```python
from build123d import *

# Parameters (mm, degrees)
EXTRUDE1_DEPTH = 0.4572
EXTRUDE2_REACH = 567.039
SKETCH2_R      = 6.35
EXTRUDE3_REACH = 567.039


with BuildPart() as part:
    # Sketch1 → Extrude1 (new body)
    with BuildSketch(Plane(origin=(0, 0, 0), x_dir=(1, 0, 0), z_dir=(0, 1, 0))):
        with BuildLine():
            Line((145.25625, 434.18125), (138.034060826, 516.73125))
            Line((138.034060826, 516.73125), (-138.034060826, 516.73125))
            Line((-138.034060826, 516.73125), (-145.25625, 434.18125))
            Line((-145.25625, 434.18125), (-228.6, 434.18125))
            Line((-228.6, 434.18125), (-228.6, 199.23125))
            Line((-228.6, 199.23125), (-145.25625, 199.23125))
            ThreePointArc((-145.25625, 199.23125), (-143.670260948, 197.712995777), (-145.117890258, 196.062290917))
            Line((-145.117890258, 196.062290917), (-223.8375, 189.175217467))
            Line((-223.8375, 189.175217467), (-223.8375, 125.149782533))
            Line((-223.8375, 125.149782533), (-145.117890258, 118.262709083))
            ThreePointArc((-145.117890258, 118.262709083), (-143.668991784, 116.653544305), (-145.173166669, 115.095925614))
            Line((-145.173166669, 115.095925614), (-228.6, 110.723710546))
            Line((-228.6, 110.723710546), (-228.6, -110.723710546))
            Line((-228.6, -110.723710546), (-145.173166669, -115.095925614))
            ThreePointArc((-145.173166669, -115.095925614), (-143.668991784, -116.653544305), (-145.117890258, -118.262709083))
            Line((-145.117890258, -118.262709083), (-223.8375, -125.149782533))
            Line((-223.8375, -125.149782533), (-223.8375, -192.356281459))
            Line((-223.8375, -192.356281459), (-145.25625, -199.23125))
            Line((-145.25625, -199.23125), (145.25625, -199.23125))
            Line((145.25625, -199.23125), (223.8375, -192.356281459))
            Line((223.8375, -192.356281459), (223.8375, -125.149782533))
            Line((223.8375, -125.149782533), (145.117890258, -118.262709083))
            ThreePointArc((145.117890258, -118.262709083), (143.668991784, -116.653544305), (145.173166669, -115.095925614))
            Line((145.173166669, -115.095925614), (228.6, -110.723710546))
            Line((228.6, -110.723710546), (228.6, 110.723710546))
            Line((228.6, 110.723710546), (145.173166669, 115.095925614))
            ThreePointArc((145.173166669, 115.095925614), (143.668991784, 116.653544305), (145.117890258, 118.262709083))
            Line((145.117890258, 118.262709083), (223.8375, 125.149782533))
            Line((223.8375, 125.149782533), (223.8375, 189.175217467))
            Line((223.8375, 189.175217467), (145.117890258, 196.062290917))
            ThreePointArc((145.117890258, 196.062290917), (143.670260948, 197.712995777), (145.25625, 199.23125))
            Line((145.25625, 199.23125), (228.6, 199.23125))
            Line((228.6, 199.23125), (228.6, 434.18125))
            Line((228.6, 434.18125), (145.25625, 434.18125))
        make_face()
    extrude(amount=EXTRUDE1_DEPTH)

    # Sketch2 → Extrude2 (cut, up to next)
    with BuildSketch(Plane(origin=(0, 0.4572, 0), x_dir=(1, 0, 0), z_dir=(0, 1, 0)), mode=Mode.PRIVATE) as extrude2_sk1:
        with Locations((-145.25625, 116.68125)):
            Circle(SKETCH2_R)
    extrude2_tool1 = extrude(extrude2_sk1.sketch, amount=-EXTRUDE2_REACH, mode=Mode.PRIVATE) & part.part
    # Sketch2 → Extrude2 (cut, up to next)
    with BuildSketch(Plane(origin=(0, 0.4572, 0), x_dir=(1, 0, 0), z_dir=(0, 1, 0)), mode=Mode.PRIVATE) as extrude2_sk2:
        with Locations((-145.25625, -116.68125)):
            Circle(SKETCH2_R)
    extrude2_tool2 = extrude(extrude2_sk2.sketch, amount=-EXTRUDE2_REACH, mode=Mode.PRIVATE) & part.part
    # Sketch2 → Extrude2 (cut, up to next)
    with BuildSketch(Plane(origin=(0, 0.4572, 0), x_dir=(1, 0, 0), z_dir=(0, 1, 0)), mode=Mode.PRIVATE) as extrude2_sk3:
        with Locations((145.25625, -116.68125)):
            Circle(SKETCH2_R)
    extrude2_tool3 = extrude(extrude2_sk3.sketch, amount=-EXTRUDE2_REACH, mode=Mode.PRIVATE) & part.part
    # Sketch2 → Extrude2 (cut, up to next)
    with BuildSketch(Plane(origin=(0, 0.4572, 0), x_dir=(1, 0, 0), z_dir=(0, 1, 0)), mode=Mode.PRIVATE) as extrude2_sk4:
        with Locations((145.25625, 116.68125)):
            Circle(SKETCH2_R)
    extrude2_tool4 = extrude(extrude2_sk4.sketch, amount=-EXTRUDE2_REACH, mode=Mode.PRIVATE) & part.part
    # Sketch2 → Extrude2 (cut, up to next)
    with BuildSketch(Plane(origin=(0, 0.4572, 0), x_dir=(1, 0, 0), z_dir=(0, 1, 0)), mode=Mode.PRIVATE) as extrude2_sk5:
        with Locations((-145.25625, 197.64375)):
            Circle(SKETCH2_R)
    extrude2_tool5 = extrude(extrude2_sk5.sketch, amount=-EXTRUDE2_REACH, mode=Mode.PRIVATE) & part.part
    # Sketch2 → Extrude2 (cut, up to next)
    with BuildSketch(Plane(origin=(0, 0.4572, 0), x_dir=(1, 0, 0), z_dir=(0, 1, 0)), mode=Mode.PRIVATE) as extrude2_sk6:
        with Locations((145.25625, 197.64375)):
            Circle(SKETCH2_R)
    extrude2_tool6 = extrude(extrude2_sk6.sketch, amount=-EXTRUDE2_REACH, mode=Mode.PRIVATE) & part.part
    add(extrude2_tool1.solids().sort_by_distance((-145.25625, 0.4572, -116.68125))[0], mode=Mode.SUBTRACT)
    add(extrude2_tool2.solids().sort_by_distance((-145.25625, 0.4572, 116.68125))[0], mode=Mode.SUBTRACT)
    add(extrude2_tool3.solids().sort_by_distance((145.25625, 0.4572, 116.68125))[0], mode=Mode.SUBTRACT)
    add(extrude2_tool4.solids().sort_by_distance((145.25625, 0.4572, -116.68125))[0], mode=Mode.SUBTRACT)
    add(extrude2_tool5.solids().sort_by_distance((-145.25625, 0.4572, -197.64375))[0], mode=Mode.SUBTRACT)
    add(extrude2_tool6.solids().sort_by_distance((145.25625, 0.4572, -197.64375))[0], mode=Mode.SUBTRACT)

    # Sketch12 → Extrude3 (cut, up to next)
    with BuildSketch(Plane(origin=(0, 0.4572, 0), x_dir=(1, 0, 0), z_dir=(0, 1, 0)), mode=Mode.PRIVATE) as extrude3_sk1:
        Polygon((-138.589613839, 510.38125), (-22.225, 510.38125), (-12.7, 516.73125), (-138.034060826, 516.73125), align=None)
    extrude3_tool1 = extrude(extrude3_sk1.sketch, amount=-EXTRUDE3_REACH, mode=Mode.PRIVATE) & part.part
    # Sketch12 → Extrude3 (cut, up to next)
    with BuildSketch(Plane(origin=(0, 0.4572, 0), x_dir=(1, 0, 0), z_dir=(0, 1, 0)), mode=Mode.PRIVATE) as extrude3_sk2:
        Polygon((12.7, 516.73125), (22.225, 510.38125), (138.589613839, 510.38125), (138.034060826, 516.73125), align=None)
    extrude3_tool2 = extrude(extrude3_sk2.sketch, amount=-EXTRUDE3_REACH, mode=Mode.PRIVATE) & part.part
    add(extrude3_tool1.solids().sort_by_distance((-77.855995, 0.4572, -513.595525))[0], mode=Mode.SUBTRACT)
    add(extrude3_tool2.solids().sort_by_distance((77.855995, 0.4572, -513.595525))[0], mode=Mode.SUBTRACT)


solid = part.part
```
Source: CAD feature listing. Evaluate the final solid. Frame: model axes, mm. Give positions to 0.01 mm unless a question says otherwise; leave off trailing zeros. Loops run counter-clockwise (first coordinate to the right, second up) from the corner with the lowest first, then second, coordinate; pieces in that order, holes last. Notation, with made-up numbers: M 15.5,-15.75 L 70.5,-15.75 A22 ccw 70.5,17.25 Z; hole C -37,-17.5 d1. An arc over 180 degrees is marked long. Put each result on its own line as item: value.
Q1. Section B-B (z = -140). Return the cut outline in (x, y).
Response values:
outline: M -223.84,0 L 223.84,0 L 223.84,0.46 L -223.84,0.46 Z
Q2. Section C-C (x = -172). Return the cut outline in (y, z), and give its area (3 significant figures).
Response values:
outline: M 0,-434.18 L 0.46,-434.18 L 0.46,-199.23 L 0,-199.23 Z; M 0,-193.71 L 0.46,-193.71 L 0.46,-120.61 L 0,-120.61 Z; M 0,-113.69 L 0.46,-113.69 L 0.46,113.69 L 0,113.69 Z; M 0,120.61 L 0.46,120.61 L 0.46,196.89 L 0,196.89 Z
area: 280 mm²
Q3. Section A-A (x = 187.5). Return the cut outline in (y, z).
Response values:
outline: M 0,-434.18 L 0.46,-434.18 L 0.46,-199.23 L 0,-199.23 Z; M 0,-192.35 L 0.46,-192.35 L 0.46,-121.97 L 0,-121.97 Z; M 0,-112.88 L 0.46,-112.88 L 0.46,112.88 L 0,112.88 Z; M 0,121.97 L 0.46,121.97 L 0.46,195.54 L 0,195.54 Z
Q4. Pin query (flat end, axial travel): P1, Ø14.5, axis at x = 145.26, z = -197.64, coming from the +Y side; P2, Ø7.5, axis at x = -145.26, z = -116.68, coming from the -Y side (3 decimals). Return the tip coordinate at first contact, or that it passes through.
Response values:
P1: stops at y = 0.46
P2: passes through
Q5. Line query: probe 1 along Z at (x, y) = (170, 0.35); probe 2 along Z at (x, y) = (-101.5, 0.25); probe 3 along X at (y, z) = (0.1, 132). Output: solid intervals per line, ascending. Write a range as [from, to].
Response values:
probe 1: z = [-434.18, -199.23], [-193.89, -120.44], [-113.79, 113.79], [120.44, 197.07]
probe 2: z = [-510.38, 199.23]
probe 3: x = [-223.84, 223.84]
